from build123d import *

# Parameters (mm, degrees)
SKETCH1_W           = 92
SKETCH1_H           = 12
BOSS_EXTRUDE1_DEPTH = 3
FILLET1_R           = 4
FILLET2_R           = 2
SKETCH2_R           = 1.4
SKETCH2_R_2         = 1.55
SKETCH2_W           = 7.5
SKETCH2_H           = 3
SKETCH2_W_2         = 5.05
CUT_EXTRUDE1_DEPTH  = 4
SKETCH3_W           = 7.5
SKETCH3_H           = 0.15
SKETCH3_W_2         = 5.05
CUT_EXTRUDE2_DEPTH  = 4


with BuildPart() as part:
    # Sketch1 → Boss-Extrude1 (new body)
    with BuildSketch(Plane(origin=(0, 0, 0), x_dir=(1, 0, 0), z_dir=(0, 1, 0))):
        with Locations((46, 6)):
            Rectangle(SKETCH1_W, SKETCH1_H)
    extrude(amount=BOSS_EXTRUDE1_DEPTH)

    # Fillet1
    fillet1_edges = [part.edges().sort_by_distance(p)[0] for p in [
        (0, 1.5, -12),
        (0, 1.5, 0),
    ]]
    fillet(fillet1_edges, radius=FILLET1_R)

    # Fillet2
    fillet2_edges = [part.edges().sort_by_distance(p)[0] for p in [
        (92, 1.5, -12),
        (92, 1.5, 0),
    ]]
    fillet(fillet2_edges, radius=FILLET2_R)

    # Sketch2 → Cut-Extrude1 (cut, through all)
    with BuildSketch(Plane(origin=(0, 3, 0), x_dir=(1, 0, 0), z_dir=(0, 1, 0))):
        with Locations((6.4, 6)):
            Circle(SKETCH2_R)
        with Locations((53.85, 6)):
            Circle(SKETCH2_R_2)
        with Locations((86, 6)):
            Circle(SKETCH2_R)
        with Locations((19.95, 6)):
            Rectangle(SKETCH2_W, SKETCH2_H)
        with Locations((73.575, 6)):
            Rectangle(SKETCH2_W_2, SKETCH2_H)
    extrude(amount=-CUT_EXTRUDE1_DEPTH, mode=Mode.SUBTRACT)

    # Sketch3 → Cut-Extrude2 (cut, through all)
    with BuildSketch(Plane(origin=(0, 3, 0), x_dir=(1, 0, 0), z_dir=(0, 1, 0))):
        with Locations((19.95, 7.575)):
            Rectangle(SKETCH3_W, SKETCH3_H)
        with Locations((19.95, 4.425)):
            Rectangle(SKETCH3_W, SKETCH3_H)
        with Locations((73.575, 7.575)):
            Rectangle(SKETCH3_W_2, SKETCH3_H)
        with Locations((73.575, 4.425)):
            Rectangle(SKETCH3_W_2, SKETCH3_H)
    extrude(amount=-CUT_EXTRUDE2_DEPTH, mode=Mode.SUBTRACT)


solid = part.part
Here's how the part is built. I have some questions about the finished solid (model axes, mm). A direction names the side the tool comes from. Round coordinates to 2 decimals unless told otherwise and drop trailing zeros. Write each loop counter-clockwise with the first axis right and the second up, starting at its lowest first coordinate (ties: lowest second). Pieces come first, ordered by that corner, then holes. Notation, with made-up numbers: (18.25, 50.5) -> (49.25, 50.5) arc R35 cw to (49.25, 88.5) -> close; hole circle Ø8 at (41, 22). An arc over 180 degrees is marked (long way). One line per item, written item: value.
1) Suppose I cut it at C-C on y = 2.55. List the corners of the cut face in (x, z) for me.
Filled sheet:
outline: (0, -8) arc R4 ccw to (4, -12) -> (90, -12) arc R2 ccw to (92, -10) -> (92, -2) arc R2 ccw to (90, 0) -> (4, 0) arc R4 ccw to (0, -4) -> close; hole circle Ø2.8 at (6.4, -6); hole (16.2, -7.65) -> (23.7, -7.65) -> (23.7, -4.35) -> (16.2, -4.35) -> close; hole circle Ø3.1 at (53.85, -6); hole (71.05, -7.65) -> (76.1, -7.65) -> (76.1, -4.35) -> (71.05, -4.35) -> close; hole circle Ø2.8 at (86, -6)
2) Suppose I cut it at B-B on x = 53.85. List the corners of the cut face in (y, z) for me.
Filled sheet:
outline: (0, -12) -> (3, -12) -> (3, -7.55) -> (0, -7.55) -> close; (0, -4.45) -> (3, -4.45) -> (3, 0) -> (0, 0) -> close
3) For faces 1 (the face through (23.7, 2, -6)), 2 (the face through (0, 1, -6)), which set-ups out of +Z, -Z, +X, -X, +Y, -Y let a thin tool reach every point of the face, with its end or its side?
Filled sheet:
face 1: +Y, -Y
face 2: +Z, -Z, -X, +Y, -Y
4) Suppose I cut it at A-A on z = -6. List the corners of the cut face in (x, y) for me.
Filled sheet:
outline: (0, 0) -> (5, 0) -> (5, 3) -> (0, 3) -> close; (7.8, 0) -> (16.2, 0) -> (16.2, 3) -> (7.8, 3) -> close; (23.7, 0) -> (52.3, 0) -> (52.3, 3) -> (23.7, 3) -> close; (55.4, 0) -> (71.05, 0) -> (71.05, 3) -> (55.4, 3) -> close; (76.1, 0) -> (84.6, 0) -> (84.6, 3) -> (76.1, 3) -> close; (87.4, 0) -> (92, 0) -> (92, 3) -> (87.4, 3) -> close
5) We'd pull the mould along Z, two halves only. Please class faces 3 (the face through (92, 1, -6)), 4 (the face through (1.141, 1.521, -10.797)), 5 (the face through (84.6, 1.52, -6.06)): released by +Z, released by -Z, zero draft, split by the parting line, or undercut.
Filled sheet:
face 3: zero draft
face 4: released by -Z
face 5: undercut
6) Suppose I cut it at D-D on x = 6.4. List the corners of the cut face in (y, z) for me.
Filled sheet:
outline: (0, -12) -> (3, -12) -> (3, -7.4) -> (0, -7.4) -> close; (0, -4.6) -> (3, -4.6) -> (3, 0) -> (0, 0) -> close
7) If I drill on line 1 (X direction, y = 1.1, z = -6); line 2 (Z direction, x = 53.85, y = 2.45); line 3 (Z direction, x = 86, y = 2.15), over which ranges is the centre line in solid material (lowest first)? Write a range as [from, to].
Filled sheet:
line 1: x = [0, 5], [7.8, 16.2], [23.7, 52.3], [55.4, 71.05], [76.1, 84.6], [87.4, 92]
line 2: z = [-12, -7.55], [-4.45, 0]
line 3: z = [-12, -7.4], [-4.6, 0]
8) I'm going to push a flat-ended pin straight in: pin 1 Ø2.5 at (x, z) = (86, -6) entering from -Y. Where does the tip first touch, or does it pass through?
Filled sheet:
pin 1: passes through
